```python
from build123d import *

# Parameters (mm, degrees)
BOSS_EXTRUDE1_DEPTH = 5
BOSS_EXTRUDE2_DEPTH = 1


with BuildPart() as part:
    # Sketch1 → Boss-Extrude1 (new body)
    with BuildSketch(Plane.XY):
        with BuildLine():
            Line((19.723160965, -30.122), (15.214660965, -41.425))
            Line((15.214660965, -41.425), (15.214660965, -45.122))
            Line((15.214660965, -45.122), (35.1855, -45.122))
            ThreePointArc((35.1855, -45.122), (42.256567812, -42.193067812), (45.1855, -35.122))
            Line((45.1855, -35.122), (45.1855, -30.122))
            Line((45.1855, -30.122), (45.1855, 35.122))
            ThreePointArc((45.1855, 35.122), (42.256567812, 42.193067812), (35.1855, 45.122))
            Line((35.1855, 45.122), (-35.1855, 45.122))
            ThreePointArc((-35.1855, 45.122), (-42.256567812, 42.193067812), (-45.1855, 35.122))
            Line((-45.1855, 35.122), (-45.1855, -30.122))
            Line((-45.1855, -30.122), (-45.1855, -35.122))
            ThreePointArc((-45.1855, -35.122), (-42.256567812, -42.193067812), (-35.1855, -45.122))
            Line((-35.1855, -45.122), (-15.086607553, -45.122))
            Line((-15.086607553, -45.122), (-15.086607553, -41.425))
            Line((-15.086607553, -41.425), (-19.722107553, -30.122))
            Line((-19.722107553, -30.122), (-24.9555, -30.122))
            ThreePointArc((-24.9555, -30.122), (-28.653668466, -28.590168466), (-30.1855, -24.892))
            Line((-30.1855, -24.892), (-30.1855, 24.892))
            ThreePointArc((-30.1855, 24.892), (-28.653668466, 28.590168466), (-24.9555, 30.122))
            Line((-24.9555, 30.122), (24.9555, 30.122))
            ThreePointArc((24.9555, 30.122), (28.653668466, 28.590168466), (30.1855, 24.892))
            Line((30.1855, 24.892), (30.1855, -24.892))
            ThreePointArc((30.1855, -24.892), (28.653668466, -28.590168466), (24.9555, -30.122))
            Line((24.9555, -30.122), (19.723160965, -30.122))
        make_face()
    extrude(amount=-BOSS_EXTRUDE1_DEPTH)

    # Sketch2 → Boss-Extrude2 (add)
    with BuildSketch(Plane.XY):
        with BuildLine():
            Line((-24.9555, 30.122), (24.9555, 30.122))
            ThreePointArc((24.9555, 30.122), (28.653668466, 28.590168466), (30.1855, 24.892))
            Line((30.1855, 24.892), (30.1855, -24.892))
            ThreePointArc((30.1855, -24.892), (28.653668466, -28.590168466), (24.9555, -30.122))
            Line((24.9555, -30.122), (19.723160965, -30.122))
            Line((19.723160965, -30.122), (15.214660965, -41.425))
            Line((15.214660965, -41.425), (15.214660965, -45.122))
            Line((15.214660965, -45.122), (35.1855, -45.122))
            ThreePointArc((35.1855, -45.122), (42.256567812, -42.193067812), (45.1855, -35.122))
            Line((45.1855, -35.122), (45.1855, 35.122))
            ThreePointArc((45.1855, 35.122), (42.256567812, 42.193067812), (35.1855, 45.122))
            Line((35.1855, 45.122), (-35.1855, 45.122))
            ThreePointArc((-35.1855, 45.122), (-42.256567812, 42.193067812), (-45.1855, 35.122))
            Line((-45.1855, 35.122), (-45.1855, -35.122))
            ThreePointArc((-45.1855, -35.122), (-42.256567812, -42.193067812), (-35.1855, -45.122))
            Line((-35.1855, -45.122), (-15.086607553, -45.122))
            Line((-15.086607553, -45.122), (-15.086607553, -41.425))
            Line((-15.086607553, -41.425), (-19.722107553, -30.122))
            Line((-19.722107553, -30.122), (-24.9555, -30.122))
            ThreePointArc((-24.9555, -30.122), (-28.653668466, -28.590168466), (-30.1855, -24.892))
            Line((-30.1855, -24.892), (-30.1855, 24.892))
            ThreePointArc((-30.1855, 24.892), (-28.653668466, 28.590168466), (-24.9555, 30.122))
        make_face()
        with BuildLine():
            Line((-19.722107553, -30.122), (-15.086607553, -41.425))
            Line((-15.086607553, -41.425), (-15.086607553, -36.275))
            Line((-15.086607553, -36.275), (15.214660965, -36.275))
            Line((15.214660965, -36.275), (15.214660965, -41.425))
            Line((15.214660965, -41.425), (19.723160965, -30.122))
            Line((19.723160965, -30.122), (24.9555, -30.122))
            ThreePointArc((24.9555, -30.122), (28.653668466, -28.590168466), (30.1855, -24.892))
            Line((30.1855, -24.892), (30.1855, 24.892))
            ThreePointArc((30.1855, 24.892), (28.653668466, 28.590168466), (24.9555, 30.122))
            Line((24.9555, 30.122), (-24.9555, 30.122))
            ThreePointArc((-24.9555, 30.122), (-28.653668466, 28.590168466), (-30.1855, 24.892))
            Line((-30.1855, 24.892), (-30.1855, -24.892))
            ThreePointArc((-30.1855, -24.892), (-28.653668466, -28.590168466), (-24.9555, -30.122))
            Line((-24.9555, -30.122), (-19.722107553, -30.122))
        make_face()
    extrude(amount=BOSS_EXTRUDE2_DEPTH)


solid = part.part
```
The listing builds one solid part. Answer for the finished solid, in the listing's coordinates (mm). A direction names the side the tool comes from. Coordinates: 2 decimals unless noted, no trailing zeros. Write each loop counter-clockwise with the first axis right and the second up, starting at its lowest first coordinate (ties: lowest second). Pieces come first, ordered by that corner, then holes. Notation, with made-up numbers: (60, 24.25) - (97, 24.25) arc R16 cw to (97, 36.25) - close; hole circle Ø8 at (-25, -18.75). An arc over 180 degrees is marked (long way). One line per item, written item: value.
1) For a pull along X with two mould halves and no side action, classify faces 4 (the flat face through (-45.186, 0, -2)), 5 (the flat face through (-1, 31, -5)), 6 (the cylindrical face through (-28.613, -28.631, -2.465)) as pulls with the +X half, pulls with the -X half, needs draft (parallel to the pull), parting line crosses it, or undercut.
Geometry check:
face 4: pulls with the -X half
face 5: needs draft
face 6: undercut
2) Find section C-C (y = -10.5). Give the vertices of the cut face in (x, z), and give its area (3 significant figures).
Geometry check:
outline: (-45.19, -5) - (-30.19, -5) - (-30.19, 0) - (30.19, 0) - (30.19, -5) - (45.19, -5) - (45.19, 1) - (-45.19, 1) - close
area: 240 mm2
3) Consider line 1 along X through (y, z) = (-8, -2.5); line 2 along Y through (x, z) = (21, -3.75); line 3 along Z through (x, y) = (28.5, 24). Determine where each line is inside the solid, lowest interval first. Write a range as from..to.
Geometry check:
line 1: x = -45.19..-30.19, 30.19..45.19
line 2: y = -45.12..-30.12, 30.12..45.12
line 3: z = 0..1
4) Find section A-A (z = -3.65). Give the vertices of the cut face in (x, y) (1 decimal), and give its area (3 significant figures).
Geometry check:
outline: (-45.2, -35.1) arc R10 ccw to (-35.2, -45.1) - (-15.1, -45.1) - (-15.1, -41.4) - (-19.7, -30.1) - (-25, -30.1) arc R5.2 cw to (-30.2, -24.9) - (-30.2, 24.9) arc R5.2 cw to (-25, 30.1) - (25, 30.1) arc R5.2 cw to (30.2, 24.9) - (30.2, -24.9) arc R5.2 cw to (25, -30.1) - (19.7, -30.1) - (15.2, -41.4) - (15.2, -45.1) - (35.2, -45.1) arc R10 ccw to (45.2, -35.1) - (45.2, 35.1) arc R10 ccw to (35.2, 45.1) - (-35.2, 45.1) arc R10 ccw to (-45.2, 35.1) - close
area: 3,950 mm2
5) Find section D-D (y = 39.5). Give the vertices of the cut face in (x, z).
Geometry check:
outline: (-44.18, -5) - (44.18, -5) - (44.18, 1) - (-44.18, 1) - close
6) Find section B-B (x = -21). Give the vertices of the cut face in (y, z).
Geometry check:
outline: (-45.12, -5) - (-30.12, -5) - (-30.12, 0) - (30.12, 0) - (30.12, -5) - (45.12, -5) - (45.12, 1) - (-45.12, 1) - close
7) This flat-tipped pin is pushed along its axis until it touches: pin 1 Ø0.5 at (x, z) = (-5.5, 0.5) entering from -Y (3 decimals). Where does it stop, or does it pass through?
Geometry check:
pin 1: stops at y = -36.275
8) A tool of negligible diameter and unlimited length cuts with its end or side. For faces 1 (the flat face through (-30.186, 0, -2)), 2 (the flat face through (15.215, -43, -2)), 3 (the flat face through (45.186, 0, -2)), from which of +Z, -Z, +X, -X, +Y, -Y can it reach the whole face along a straight path? Write none if from no direction.
Geometry check:
face 1: -Z
face 2: +Z, -Z, -Y
face 3: +Z, -Z, +X, +Y, -Y
